Check sheet for the modelled part. Datum: model origin and axes. Units: mm. A direction names the side the tool comes from. Round coordinates to 2 decimals unless told otherwise and drop trailing zeros. Loops run counter-clockwise (first coordinate to the right, second up) from the corner with the lowest first, then second, coordinate; pieces in that order, holes last. Notation, with made-up numbers: (77, 22.25) - (128, 22.25) arc R23 ccw to (128, 39.25) - close; hole circle Ø6 at (-23.5, 41.5). An arc over 180 degrees is marked (long way). Answer in a Markdown table with one row per item. Add a question column.
(1) Cross-section at C-C on y = -22. Enter the section's corners in (x, z).
(2) Cross-section at A-A on x = -6. Enter the section's corners in (y, z), then the cut area to 3 significant figures.
(3) Cross-section at D-D on x = -64. Enter the section's corners in (y, z), then the cut area to 3 significant figures.
(4) Thickness scan on line 1 along Y through (x, z) = (-47.5, -14); line 2 along Y through (x, z) = (8, -30); line 3 along X through (y, z) = (-116.5, -47.5). Record the ranges inside material, lowest first.
(5) Access from +Z, -Z, +X, -X, +Y, -Y to the whole of each face (thin tool, end or side, straight path). Record for faces 1 (the cylindrical face through (-33.03, -60, -0.95)), 2 (the flat face through (2.949, -89, 32)), 3 (the cylindrical face through (16.79, -49.27, 61.59)).
(6) Cross-section at B-B on y = -83. Enter the section's corners in (x, z).
(7) Mould release check, pull along Y, two halves, no side actions. Record for faces 4 (the cylindrical face through (103.1, -25.684, -62.437)), 5 (the cylindrical face through (66.06, -49.27, 10.34)), 6 (the cylindrical face through (-67.962, -76.735, 0.425)), 7 (the cylindrical face through (103.02, -1.45, -49.44)): +Y half, -Y half, draft (parallel to the pull), parting line (faces both ways), or undercut.
(8) Gauge pin test, flat ends, axial feed: pin 1 (2.5 mm diameter, centred on y = -57, z = -26, fed in from +X); pin 2 (22.5 mm diameter, centred on x = -10.5, y = -97, fed in from -Z); pin 3 (1.5 mm diameter, centred on x = 80, z = -20.5, fed in from -Y). Record the tip position at first contact, or that the pin passes through.
from build123d import *

# Parameters (mm, degrees)
F0_W     = 203.2
F0_H     = 127
F1_DEPTH = 127
F3_DEPTH = 76.2
F4_SIZE2 = 101.6
F4_SIZE  = 76.2
F5_R     = 5.08
F6_R     = 15.24
F7_DEPTH = 50.8
F8_R     = 20.5391892085
F9_DEPTH = 127


with BuildPart() as f1:
    # F0 (on Front) → F1 (new body)
    with BuildSketch(Plane.XZ):
        with Locations((2.9485966027, -0.464142194)):
            Rectangle(F0_W, F0_H)
    extrude(amount=F1_DEPTH)

    # F2 (on face) → F3 (cut)
    with BuildSketch(Plane.XZ.offset(127)):
        Polygon((-35.1514033973, 0), (-35.1514033973, -63.964142194), (104.5485966027, -63.964142194), (104.5485966027, 63.035857806), (2.9485966027, 63.035857806), (2.9485966027, 0), align=None)
    extrude(amount=-F3_DEPTH, mode=Mode.SUBTRACT)

    # F4
    f4_edges = [f1.edges().sort_by_distance(p)[0] for p in [
        (104.548597, -25.4, 63.035858),
    ]]
    f4_side = f1.faces().sort_by_distance((-18.822832, -52.614286, 63.035858))[0]
    chamfer(f4_edges, length=F4_SIZE, length2=F4_SIZE2, reference=f4_side)

    # F5
    f5_edges = [f1.edges().sort_by_distance(p)[0] for p in [
        (-98.651403, -63.5, 63.035858),
        (-47.851403, -127, 63.035858),
        (2.948597, -88.9, 63.035858),
        (15.648597, -50.8, 63.035858),
        (28.348597, -25.4, 63.035858),
        (-35.151403, 0, 63.035858),
        (2.948597, -127, 31.517929),
        (2.948597, -88.9, 0),
        (-35.151403, -127, -31.982071),
        (-16.101403, -127, 0),
        (-16.101403, -50.8, 0),
        (-35.151403, -88.9, 0),
        (-35.151403, -50.8, -31.982071),
        (-66.901403, -127, -63.964142),
        (-35.151403, -88.9, -63.964142),
        (34.698597, -50.8, -63.964142),
        (104.548597, -25.4, -63.964142),
        (104.548597, -50.8, -51.264142),
        (104.548597, 0, -51.264142),
        (104.548597, -25.4, -38.564142),
        (66.448597, 0, 12.235858),
        (66.448597, -50.8, 12.235858),
        (-98.651403, 0, -0.464142),
        (2.948597, 0, -63.964142),
        (-98.651403, -63.5, -63.964142),
        (-98.651403, -127, -0.464142),
        (2.948597, -50.8, 31.517929),
    ]]
    fillet(f5_edges, radius=F5_R)

    # F6 (on face) → F7 (cut, through all)
    with BuildSketch(Plane.XZ.offset(50.8)):
        with Locations((20.7285966027, -18.244142194)):
            Circle(F6_R)
    extrude(amount=-F7_DEPTH, mode=Mode.SUBTRACT)

    # F8 (on face) → F9 (cut, through all)
    with BuildSketch(Plane.XY.offset(63.035857806)):
        with Locations((-47.4430248141, -77.6382982731)):
            Circle(F8_R)
    extrude(amount=-F9_DEPTH, mode=Mode.SUBTRACT)


solid = f1.part
Answers:
| question | item | result |
|---|---|---|
| 1 | outline | (-98.65, -58.88) arc R5.08 ccw to (-93.57, -63.96) - (99.47, -63.96) arc R5.08 ccw to (104.55, -58.88) - (104.55, -40.26) arc R5.08 ccw to (103.53, -37.21) - (29.87, 61) arc R5.08 ccw to (25.81, 63.04) - (-93.57, 63.04) arc R5.08 ccw to (-98.65, 57.96) - close; hole circle Ø30.48 at (20.73, -18.24) |
| 2 | outline | (-127, 5.08) arc R5.08 ccw to (-121.92, 0) - (-55.88, 0) arc R5.08 cw to (-50.8, -5.08) - (-50.8, -58.88) arc R5.08 ccw to (-45.72, -63.96) - (-5.08, -63.96) arc R5.08 ccw to (0, -58.88) - (0, 57.96) arc R5.08 ccw to (-5.08, 63.04) - (-121.92, 63.04) arc R5.08 ccw to (-127, 57.96) - close |
| 2 | area | 11,200 mm^2 |
| 3 | outline | (-127, -58.88) arc R5.08 ccw to (-121.92, -63.96) - (-89.79, -63.96) - (-89.79, 63.04) - (-121.92, 63.04) arc R5.08 ccw to (-127, 57.96) - close; (-65.48, -63.96) - (-5.08, -63.96) arc R5.08 ccw to (0, -58.88) - (0, 57.96) arc R5.08 ccw to (-5.08, 63.04) - (-65.48, 63.04) - close |
| 3 | area | 13,000 mm^2 |
| 4 | line 1 | y = -127 to -98.18, -57.1 to 0 |
| 4 | line 2 | y = -50.8 to 0 |
| 4 | line 3 | x = -98.65 to -35.15 |
| 5 | face 1 | -Z, +X, -Y |
| 5 | face 2 | +Z, -Z, +X, -Y |
| 5 | face 3 | +Z, +X, -Y |
| 6 | outline | (-98.65, -58.88) arc R5.08 ccw to (-93.57, -63.96) - (-67.27, -63.96) - (-67.27, 63.04) - (-93.57, 63.04) arc R5.08 ccw to (-98.65, 57.96) - close; (-27.62, 0) - (-2.13, 0) arc R5.08 ccw to (2.95, 5.08) - (2.95, 57.96) arc R5.08 ccw to (-2.13, 63.04) - (-27.62, 63.04) - close |
| 7 | face 4 | draft |
| 7 | face 5 | -Y half |
| 7 | face 6 | undercut |
| 7 | face 7 | +Y half |
| 8 | pin 1 | stops at x = -35.15 |
| 8 | pin 2 | stops at z = 0 |
| 8 | pin 3 | stops at y = -50.8 |
